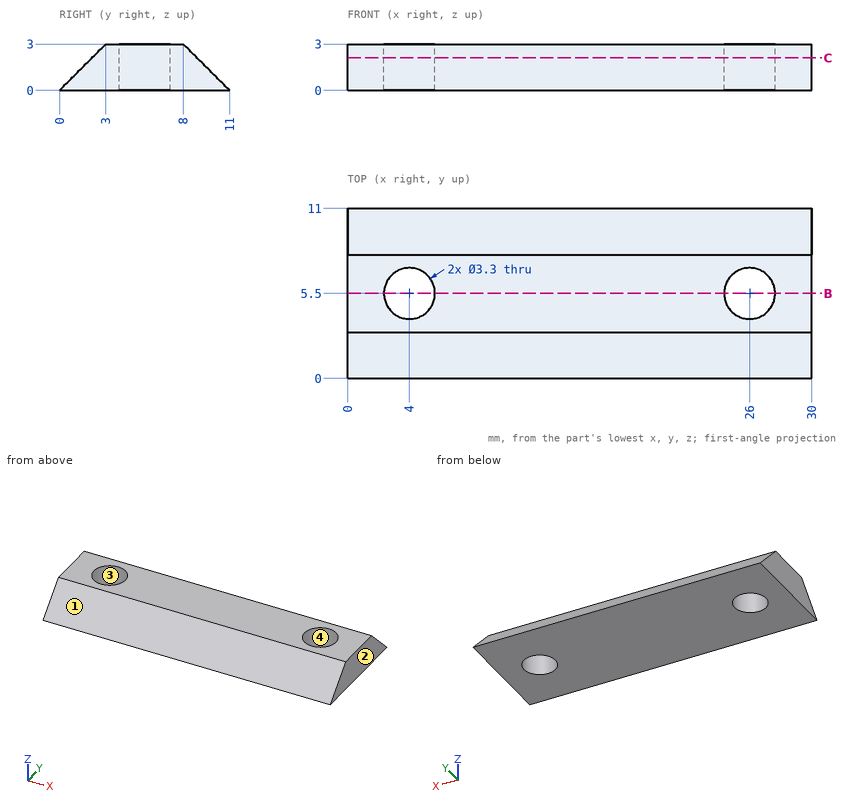
Geometry check sheet. Reference: drawing and pictorial views, mm from the part's lowest x, y, z. Round coordinates to 2 decimals unless told otherwise and drop trailing zeros. Write each loop counter-clockwise with the first axis right and the second up, starting at its lowest first coordinate (ties: lowest second). Pieces come first, ordered by that corner, then holes.
1. Scan lines: L1, parallel to X at y = 5.5, z = 1.05; L2, parallel to X at y = 6.25, z = 1.6; L3, parallel to Y at x = 27.25, z = 0.8. Record each from-to range of solid material in increasing order.
2. Section check B-B on y = 5.5. Enter the section's corners in (x, z), plus the area to 3 significant figures.
3. Section check C-C on z = 2.1. Enter the section's corners in (x, y).
4. Draft check along Y on the marked faces 1, 2, 3 and 4. Enter one of: +Y half, -Y half, draft (parallel to the pull), parting line (faces both ways), or undercut.
5. Gauge pin test, flat ends, axial feed: P1, Ø1, axis at x = 16.5, z = 1.5, coming from the +Y side; P2, Ø1.5, axis at x = 19, z = 0.5, coming from the -Y side. Record the tip position at first contact, or that the pin passes through.
Answer:
1. L1: x = 0 to 2.35, 5.65 to 24.35, 27.65 to 30
1. L2: x = 0 to 2.53, 5.47 to 24.53, 27.47 to 30
1. L3: y = 0.8 to 4.42, 6.58 to 10.2
2. outline: (0, 0) - (2.35, 0) - (2.35, 3) - (0, 3) - close; (5.65, 0) - (24.35, 0) - (24.35, 3) - (5.65, 3) - close; (27.65, 0) - (30, 0) - (30, 3) - (27.65, 3) - close
2. area: 70.2 mm2
3. outline: (0, 2.1) - (30, 2.1) - (30, 8.9) - (0, 8.9) - close; hole circle Ø3.3 at (4, 5.5); hole circle Ø3.3 at (26, 5.5)
4. face 1: -Y half
4. face 2: draft
4. face 3: undercut
4. face 4: undercut
5. P1: stops at y = 10
5. P2: stops at y = 0
